Geometry check sheet. Reference: the model listing, model coordinates, mm. Coordinates: 2 decimals unless noted, no trailing zeros. Order: outer loops, then holes, each group sorted by start corner. A loop starts at its lowest first (then second) coordinate and runs counter-clockwise, first axis right, second up. Notation, with made-up numbers: M 75.25,1 L 103.25,1 A17 cw 103.25,20 Z; hole C 62,-22.5 d9. An arc over 180 degrees is marked long. One line per item, written item: value. Start each with the question number.
1) Draft check along Y on faces 1 (the flat face through (-104, -7, -38.1)), 2 (the cylindrical face through (110.12, 495.92, 0.44)), 3 (the cylindrical face through (13.77, 61.99, -0.53)). Enter one of: pulls with the +Y half, pulls with the -Y half, needs draft (parallel to the pull), parting line crosses it, or undercut.
2) Sectioned sample at C-C, the plane z = 14.5. Enter the section's corners in (x, y).
3) Go/stop test with flat-tipped pins: P1, Ø5, axis at x = 193, z = -16, coming from the -Y side; P2, Ø1, axis at y = 219.5, z = 22, coming from the +X side; P3, Ø5, axis at x = -381.5, z = -26.5, coming from the -Y side. Record where each tip stops, or that it passes through.
4) Sectioned sample at A-A, the plane y = 0. Enter the section's corners in (x, z).
5) Sectioned sample at B-B, the plane x = 0. Enter the section's corners in (y, z).
6) Thickness scan on L1, parallel to Y at x = 0, z = 0; L2, parallel to X at y = 331, z = 2.5; L3, parallel to X at y = -458, z = -1.5. Record the ranges inside material, lowest first. Write a range as from..to.
```python
from build123d import *

# Parameters (mm, degrees)
SKETCH1_R           = 508
SKETCH1_R_2         = 63.5
SKETCH1_R_3         = 50.8
BOSS_EXTRUDE1_DEPTH = 38.1
FILLET1_R           = 6.35


with BuildPart() as part:
    # Sketch1 → Boss-Extrude1 (new, symmetric)
    with BuildSketch(Plane.XY):
        with Locations(Location((0, 0, 0), (0, 0, 180))):
            Circle(SKETCH1_R)
        with Locations(Location((0, 0, 0), (0, 0, 180))):
            Circle(SKETCH1_R_2, mode=Mode.SUBTRACT)
        with Locations(Location((0, 355.6, 0), (0, 0, 180))):
            Circle(SKETCH1_R_3, mode=Mode.SUBTRACT)
    extrude(amount=BOSS_EXTRUDE1_DEPTH, both=True)

    # Fillet1
    fillet1_edges = [part.edges().sort_by_distance(p)[0] for p in [
        (508, 0, -38.1),
        (508, 0, 38.1),
    ]]
    fillet(fillet1_edges, radius=FILLET1_R)


solid = part.part
```
Final values:
1. face 1: needs draft
1. face 2: parting line crosses it
1. face 3: undercut
2. outline: C 0,0 d1016; hole C 0,0 d127; hole C 0,355.6 d101.6
3. P1: stops at y = -470.93
3. P2: stops at x = 458.37
3. P3: stops at y = -338.26
4. outline: M -508,-31.75 A6.35 ccw -501.65,-38.1 L -63.5,-38.1 L -63.5,38.1 L -501.65,38.1 A6.35 ccw -508,31.75 Z; M 63.5,-38.1 L 501.65,-38.1 A6.35 ccw 508,-31.75 L 508,31.75 A6.35 ccw 501.65,38.1 L 63.5,38.1 Z
5. outline: M -508,-31.75 A6.35 ccw -501.65,-38.1 L -63.5,-38.1 L -63.5,38.1 L -501.65,38.1 A6.35 ccw -508,31.75 Z; M 63.5,-38.1 L 304.8,-38.1 L 304.8,38.1 L 63.5,38.1 Z; M 406.4,-38.1 L 501.65,-38.1 A6.35 ccw 508,-31.75 L 508,31.75 A6.35 ccw 501.65,38.1 L 406.4,38.1 Z
6. L1: y = -508..-63.5, 63.5..304.8, 406.4..508
6. L2: x = -385.36..-44.45, 44.45..385.36
6. L3: x = -219.77..219.77
